```python
from build123d import *

# Parameters (mm, degrees)
F1_W     = 1000
F1_H     = 364.5
F1_R     = 40
F2_DEPTH = 19


with BuildPart() as f2:
    # F1 (on Front) → F2 (new body)
    with BuildSketch(Plane.XZ):
        with Locations((500, 207.25)):
            Rectangle(F1_W, F1_H)
        with Locations((80, 105)):
            Circle(F1_R, mode=Mode.SUBTRACT)
    extrude(amount=F2_DEPTH)


with BuildPart() as f2_1:
    # F3: moved
    add(f2.part.moved(Location((0, 0, -25))))


solid = f2_1.part
```
CAD build for the part. Positions are in the model's coordinates, mm. Coordinates: 2 decimals unless noted, no trailing zeros. Order: outer loops, then holes, each group sorted by start corner. A loop starts at its lowest first (then second) coordinate and runs counter-clockwise, first axis right, second up.
(1) Saw through at B-B, the plane z = 80. Write the cut outline in (x, y).
Solution:
outline: (0, -19) - (40, -19) - (40, 0) - (0, 0) - close; (120, -19) - (1000, -19) - (1000, 0) - (120, 0) - close
(2) Mould opens along Z. For faces 1 (the face through (493, -9, 364.5)), 2 (the face through (1000, -9, 180)), 3 (the face through (493, -9, 0)), 4 (the face through (118.153, -9.367, 92.015)) say: released by +Z, released by -Z, zero draft, split by the parting line, or undercut.
Solution:
face 1: released by +Z
face 2: zero draft
face 3: released by -Z
face 4: undercut
(3) Drill centre lines: L1, parallel to Z at x = 80, y = -6.5; L2, parallel to X at y = -14.5, z = 79.5; L3, parallel to X at y = -6.75, z = 50. Where is each one in solid material? Low to high.
Solution:
L1: z = 0 to 40, 120 to 364.5
L2: x = 0 to 40, 120 to 1000
L3: x = 0 to 53.54, 106.46 to 1000
(4) Saw through at A-A, the plane x = 80. Write the cut outline in (y, z).
Solution:
outline: (-19, 0) - (0, 0) - (0, 40) - (-19, 40) - close; (-19, 120) - (0, 120) - (0, 364.5) - (-19, 364.5) - close
